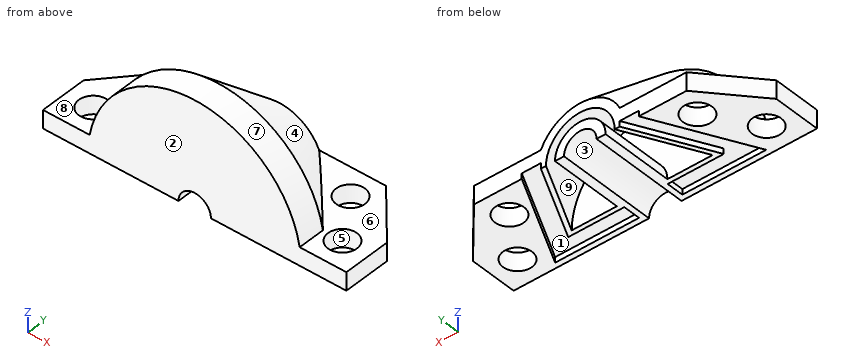
from build123d import *

# Parameters (mm, degrees)
SKETCH1_W             = 1
SKETCH1_H             = 8
REVOLVE1_ANGLE        = 180
SKETCH2_R             = 1.6
BOSS_EXTRUDE1_DEPTH   = 2
BOSS_EXTRUDE1_2_DEPTH = 2
REVOLVE2_ANGLE        = 180
CUT_EXTRUDE1_DEPTH    = 0.6


with BuildPart() as part:
    # Sketch1 → Revolve1 (revolve)
    with BuildSketch(Plane.XY):
        Polygon((-1.8, -3), (-1.8, 0), (-2.8, 0), (-7.8, 0), (-10.8, 0), (-10.8, -3), align=None)
        Polygon((-10.8, 0), (-3.8, 8), (-7.8, 0), align=None)
        with Locations((-2.3, 4)):
            Rectangle(SKETCH1_W, SKETCH1_H)
    revolve(axis=Axis((0, 0, 0), (0, 1, 0)), revolution_arc=REVOLVE1_ANGLE)



with BuildPart() as body_2:
    # Sketch2 → Boss-Extrude1 (new body)
    with BuildSketch(Plane(origin=(0, 0, 0), x_dir=(-1, 0, 0), z_dir=(0, 0, -1))):
        Polygon((-10.8, -3), (-16.8, -3), (-16.8, 2.254410697), (-11.77260936, 8), (-3.8, 8), (-10.8, 0), align=None)
        with Locations((-10.41130468, 5)):
            Circle(SKETCH2_R, mode=Mode.SUBTRACT)
        with Locations((-13.8, 0)):
            Circle(SKETCH2_R, mode=Mode.SUBTRACT)
    extrude(amount=-BOSS_EXTRUDE1_DEPTH)


with BuildPart() as body_3:
    # Sketch2 → Boss-Extrude1 2 (new body)
    with BuildSketch(Plane(origin=(0, 0, 0), x_dir=(-1, 0, 0), z_dir=(0, 0, -1))):
        Polygon((10.8, 0), (3.8, 8), (11.77260936, 8), (16.8, 2.254410697), (16.8, -3), (10.8, -3), align=None)
        with Locations(Location((13.8, 0, 0), (0, 0, 180))):
            Circle(SKETCH2_R, mode=Mode.SUBTRACT)
        with Locations(Location((10.41130468, 5, 0), (0, 0, 180))):
            Circle(SKETCH2_R, mode=Mode.SUBTRACT)
    extrude(amount=-BOSS_EXTRUDE1_2_DEPTH)


with BuildPart() as part_1:
    add(part.part)

    add(body_2.part)  # Revolve2 merges body 2

    add(body_3.part)  # Revolve2 merges body 3
    # Sketch3 → Revolve2 (revolve)
    with BuildSketch(Plane(origin=(0, 0, 0), x_dir=(-1, 0, 0), z_dir=(0, 0, -1))):
        Polygon((-11.8, -3), (-11.8, 0), (-4.8, 8), (-3.8, 8), (-10.8, 0), (-10.8, -3), align=None)
    revolve(axis=Axis((0, 0, 0), (0, -1, 0)), revolution_arc=REVOLVE2_ANGLE)

    # Sketch4 → Cut-Extrude1 (cut)
    with BuildSketch(Plane(origin=(0, 0, 0), x_dir=(-1, 0, 0), z_dir=(0, 0, -1))):
        Polygon((-6.483281573, 8), (-11.683281573, -2.4), (-2.4, -2.4), (-2.4, -0.5), (-8.609016994, -0.5), (-4.359016994, 8), align=None)
        Polygon((2.4, -2.4), (11.683281573, -2.4), (6.383281573, 8.2), (4.259016994, 8.2), (8.609016994, -0.5), (2.4, -0.5), align=None)
    extrude(amount=-CUT_EXTRUDE1_DEPTH, mode=Mode.SUBTRACT)


solid = part_1.part
For this review, take the finished solid that the model builds, in its own axes (mm). Face numbers are marked on the shaded views. A direction names the side the tool comes from. Give positions to 0.01 mm unless a question says otherwise; leave off trailing zeros. Order: outer loops, then holes, each group sorted by start corner. A loop starts at its lowest first (then second) coordinate and runs counter-clockwise, first axis right, second up. Notation, with made-up numbers: M 80,10.25 L 128,10.25 A19 cw 128,15.25 Z; hole C 87,29 d8. An arc over 180 degrees is marked long. Answer in a Markdown table with one row per item. Add a question column.
(1) Consider section C-C on x = 0. State the section outline as (y, z) points.
(2) Mouldability with a two-part tool opening along Y and no side actions: class the marked faces 1, 2, 3 and 4 as +Y half, -Y half, draft (parallel to the pull), parting line (faces both ways), or undercut.
(3) For the marked faces 5, 6, 7, 8 and 9, list the 3-axis set-ups (+Z, -Z, +X, -X, +Y, -Y) from which the entire face can be reached by the end or side of a thin tool; tool diameter is ignored.
(4) Wall thickness on probe 1 along Y at (x, z) = (-10.5, 1.75); probe 2 along X at (y, z) = (1.25, 1.5); probe 3 along Z at (x, y) = (10, 7.5): over which ranges is each line inside the solid? List them lowest first. Write a range as [from, to].
(5) Consider section B-B on z = 1. Give the number of separate pieces and of enclosed holes in the cut face, and give its area (3 significant figures).
(6) Consider section A-A on x = -13.8. State the section outline as (y, z) points, and give its area (3 significant figures).
(7) For pin 1 (4.5 mm diameter, centred on x = -6, y = 1, fed in from -Z); pin 2 (5 mm diameter, centred on x = -2.5, y = 6.5, fed in from +Z); pin 3 (5.5 mm diameter, centred on x = 8, y = 2, fed in from +Z); pin 4 (3 mm diameter, centred on x = -13.8, y = 0, fed in from -Z), all flat-tipped, find the tip position at first contact; note any pin that passes through.
Evaluation:
| question | item | result |
|---|---|---|
| 1 | outline | M -3,1.8 L 8,1.8 L 8,2.8 L 0,2.8 L 0,7.8 L 8,3.8 L 8,4.8 L 0,11.8 L -3,11.8 Z |
| 2 | face 1 | undercut |
| 2 | face 2 | -Y half |
| 2 | face 3 | draft |
| 2 | face 4 | +Y half |
| 3 | face 5 | +Z, -Z |
| 3 | face 6 | +Z, +X, +Y |
| 3 | face 7 | +Z, +Y, -Y |
| 3 | face 8 | +Z, -X, +Y |
| 3 | face 9 | none |
| 4 | probe 1 | y = [-3, 3.4], [6.6, 8] |
| 4 | probe 2 | x = [-16.8, -14.8], [-12.8, -7.02], [-2.36, -0.99], [0.99, 2.36], [7.02, 12.8], [14.8, 16.8] |
| 4 | probe 3 | z = [0, 2] |
| 5 | separate pieces | 2 |
| 5 | enclosed holes | 4 |
| 5 | area | 226 mm^2 |
| 6 | outline | M -3,0 L -1.6,0 L -1.6,2 L -3,2 Z; M 1.6,0 L 5.68,0 L 5.68,2 L 1.6,2 Z |
| 6 | area | 11.0 mm^2 |
| 7 | pin 1 | stops at z = 0 |
| 7 | pin 2 | stops at z = 8.01 |
| 7 | pin 3 | stops at z = 10.09 |
| 7 | pin 4 | passes through |
